from build123d import *

# Parameters (mm, degrees)
SKETCH2_R           = 3
BOSS_EXTRUDE1_DEPTH = 5
THREAD1_PITCH       = 1


with BuildPart() as part:
    # Sketch2 → Boss-Extrude1 (new body)
    with BuildSketch(Plane.XY):
        with BuildLine():
            Line((-57, -15), (57, -15))
            ThreePointArc((57, -15), (59.121320344, -14.121320344), (60, -12))
            Line((60, -12), (60, 12))
            ThreePointArc((60, 12), (59.121320344, 14.121320344), (57, 15))
            Line((57, 15), (-57, 15))
            ThreePointArc((-57, 15), (-59.121320344, 14.121320344), (-60, 12))
            Line((-60, 12), (-60, -12))
            ThreePointArc((-60, -12), (-59.121320344, -14.121320344), (-57, -15))
        make_face()
        Circle(SKETCH2_R, mode=Mode.SUBTRACT)
    extrude(amount=BOSS_EXTRUDE1_DEPTH)

    # Thread1: the profile of Thread Profile2 profile screwed along a right-hand helix of 5 turns, 8 arcs to a turn; built about Z, then put on its axis
    thread1_z = Axis((0, 0, 0), (0, 0, 1))
    thread1_corners = [(3.0003, 0, -0.000173205), (3.0003, 0, 0.700173203), (2.5669873, 0, 0.449999999), (2.5669873, 0, 0.249999999)]
    with BuildLine(mode=Mode.PRIVATE) as thread1_profile:
        Line(thread1_corners[0], thread1_corners[1])
        Line(thread1_corners[1], thread1_corners[2])
        Line(thread1_corners[2], thread1_corners[3])
        Line(thread1_corners[3], thread1_corners[0])
    thread1_cap = Face(thread1_profile.wire())
    thread1_turn_angles = [0, 22.5, 45, 67.5, 90, 112.5, 135, 157.5, 180, 202.5, 225, 247.5, 270, 292.5, 315, 337.5, 360]
    thread1_turn_weights = [1, 0.9238795325112867, 1, 0.9238795325112867, 1, 0.9238795325112867, 1, 0.9238795325112867, 1, 0.9238795325112867, 1, 0.9238795325112867, 1, 0.9238795325112867, 1, 0.9238795325112867, 1]
    thread1_turn_rails = [Edge.make_bspline([Vector(p[0], p[1], 0).rotate(thread1_z, thread1_turn_angles[k]) / thread1_turn_weights[k] + Vector(0, 0, p[2] + THREAD1_PITCH * thread1_turn_angles[k] / 360) for k in range(17)], [0, 0, 0, 1, 1, 2, 2, 3, 3, 4, 4, 5, 5, 6, 6, 7, 7, 8, 8, 8], 2, thread1_turn_weights) for p in thread1_corners]
    thread1_turn_sides = [Face.make_surface_from_curves(thread1_turn_rails[p[0]], thread1_turn_rails[p[1]]) for p in [(0, 1), (1, 2), (2, 3), (3, 0)]]
    thread1 = Plane(origin=(0, 0, 0), x_dir=(1, 0, 0), z_dir=(0, 0, 1)) * Solid(Shell([*[p.moved(Location((0, 0, THREAD1_PITCH * i))) for i in range(5) for p in thread1_turn_sides], thread1_cap, thread1_cap.rotate(thread1_z, 1800).moved(Location((0, 0, THREAD1_PITCH * 1800 / 360)))]))
    add(thread1)


solid = part.part
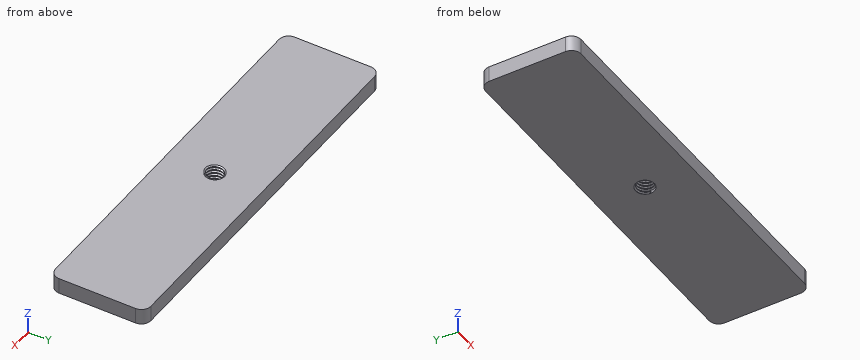
Input: part model. Units: mm. Frame: model coordinates. Give positions to 0.01 mm unless a question says otherwise; leave off trailing zeros. Order: outer loops, then holes, each group sorted by start corner. A loop starts at its lowest first (then second) coordinate and runs counter-clockwise, first axis right, second up. Notation, with made-up numbers: (22, 54.5) - (28, 54.5) arc R18 cw to (28, 79.5) - close; hole circle Ø11 at (46, 33.5). An arc over 180 degrees is marked (long way). Answer as a JSON object with one key per item and string values. Group by question number.
Q1. First-contact query: pin 1 Ø5 at (x, y) = (0, 0) entering from -Z; pin 2 Ø4 at (x, y) = (-32.5, -9) entering from +Z; pin 3 Ø5.5 at (x, y) = (0, 0) entering from -Z. Flat tips, straight axial feed; report the tip coordinate or a pass-through.
Q2. Cut plane B-B, the plane y = 10. Output: boundary loops of the cut face in (x, z), then the cut area to 3 significant figures.
Q3. Line query: probe 1 along Y at (x, z) = (0, 4.6); probe 2 along X at (y, z) = (0, 0.75). Output: solid intervals per line, ascending.
Q4. Cut plane A-A, the plane x = 20.5. Output: boundary loops of the cut face in (y, z).
Results:
{
 "1": {"pin 1": "through", "pin 2": "z = 5", "pin 3": "z = 0.14"},
 "2": {"outline": "(-60, 0) - (60, 0) - (60, 5) - (-60, 5) - close", "area": "600 mm^2"},
 "3": {"probe 1": "-15 to -3, 2.57 to 15", "probe 2": "-60 to -2.57, 3 to 60"},
 "4": {"outline": "(-15, 0) - (15, 0) - (15, 5) - (-15, 5) - close"}
}
